Study the drawing (mm; zero at the part's minimum x, y, z) and answer. Round coordinates to 2 decimals unless told otherwise and drop trailing zeros. Loops run counter-clockwise (first coordinate to the right, second up) from the corner with the lowest first, then second, coordinate; pieces in that order, holes last. Notation, with made-up numbers: M 79.5,75.25 L 105.5,75.25 A23 cw 105.5,87.25 Z; hole C 49.25,32 d7. An arc over 180 degrees is marked long. Put each result on its own line as item: value. Start each with the question number.
(1) Section A-A, the plane x = 220 is taken. Determine the outline of the cut face in (y, z).
(2) Flat-ended cylindrical pins translate along their axes: P1, Ø2, axis at x = 164, z = 395, coming from the -Y side; P2, Ø2.5, axis at x = 106.5, y = 2.5, coming from the +Z side; P3, Ø3, axis at x = 382.5, y = 1, coming from the +Z side; P4, Ø2.5, axis at y = 2, z = 331.5, coming from the +X side. Find the tip coordinate at first contact, or state that the pin passes through.
(3) Straight lines are drawn through the part: line 1 (Z direction, x = 101.5, y = 3.85) (1 decimal); line 2 (Z direction, x = 219.5, y = 0.8). For each, find the intervals that lie inside material, in ascending order.
(4) Section B-B, the plane z = 220 is taken. Determine the outline of the cut face in (x, y), then the cut area to 3 significant figures.
(5) Section C-C, the plane x = 343 is taken. Determine the outline of the cut face in (y, z), then the cut area to 3 significant figures.
(6) Section D-D, the plane y = 1.35 is taken. Count the separate pieces of the cut face and the enclosed holes in it, then the cut area to 3 significant figures.
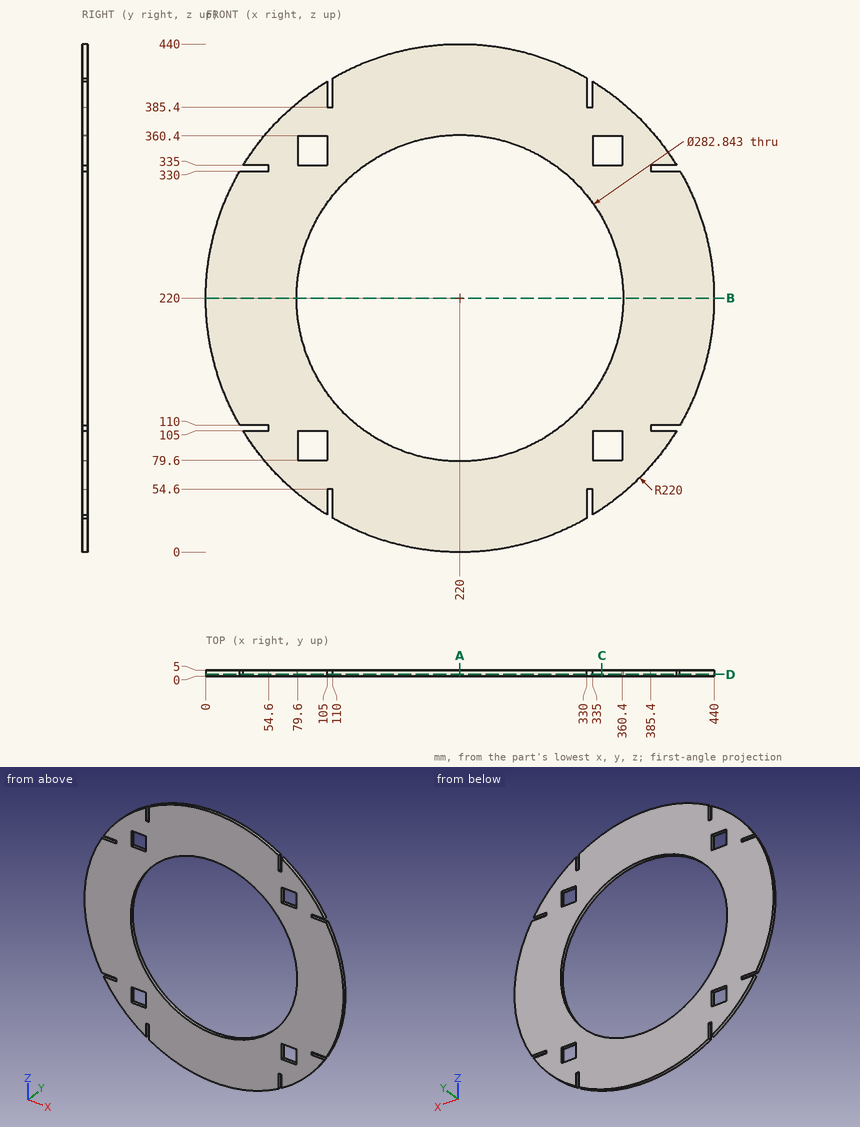
Recorded:
1. outline: M 0,0 L 5,0 L 5,78.58 L 0,78.58 Z; M 0,361.42 L 5,361.42 L 5,440 L 0,440 Z
2. P1: stops at y = 0
2. P2: stops at z = 385.4
2. P3: stops at z = 369.93
2. P4: stops at x = 385.4
3. line 1: z = 34.6 to 79.6, 105 to 142.8, 297.2 to 335, 360.4 to 405.4
3. line 2: z = 0 to 78.58, 361.42 to 440
4. outline: M 0,0 L 78.58,0 L 78.58,5 L 0,5 Z; M 361.42,0 L 440,0 L 440,5 L 361.42,5 Z
4. area: 786 mm²
5. outline: M 0,37.6 L 5,37.6 L 5,79.6 L 0,79.6 Z; M 0,105 L 5,105 L 5,150.21 L 0,150.21 Z; M 0,289.79 L 5,289.79 L 5,335 L 0,335 Z; M 0,360.4 L 5,360.4 L 5,402.4 L 0,402.4 Z
5. area: 872 mm²
6. separate pieces: 1
6. enclosed holes: 5
6. area: 85,700 mm²
